Can you work these out from the drawing? Everything is in mm from the part's minimum corner. Round coordinates to 2 decimals unless told otherwise and drop trailing zeros. Loops run counter-clockwise (first coordinate to the right, second up) from the corner with the lowest first, then second, coordinate; pieces in that order, holes last. Notation, with made-up numbers: (27.5, 53) - (66.5, 53) arc R13 ccw to (66.5, 58) - close; hole circle Ø9 at (-38.75, -20). An arc over 180 degrees is marked (long way). Put each result on its own line as item: value. Start each with the question number.
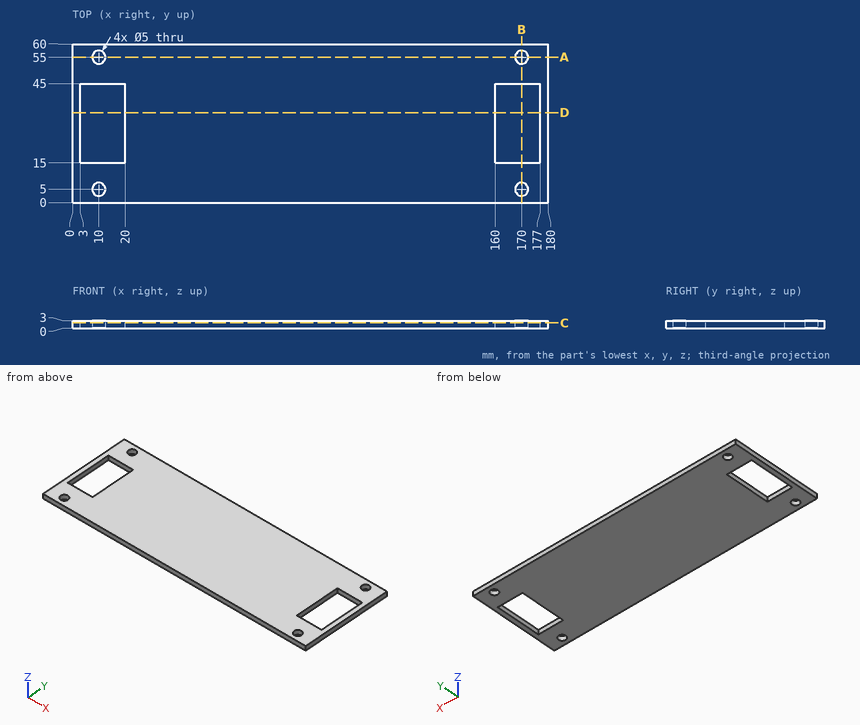
Item 1: Will this pin go through, and if not, where does the flat tip stop? P1, Ø4.5, axis at x = 170, y = 55, coming from the +Z side (3 decimals).
Item 2: I need wall thicknesses on line 1 (X direction, y = 19, z = 1.05); line 2 (Y direction, x = 170, z = 1.1); line 3 (X direction, y = 4, z = 0.85). Which ranges of each line are inside material? Lowest first, please. Write a range as from..to.
Item 3: Suppose I cut it at C-C, the plane z = 2.1. List the corners of the cut face in (x, y) for me, then the cut area to 3 significant figures.
Item 4: Suppose I cut it at D-D, the plane y = 34. List the corners of the cut face in (x, z) for me.
Item 5: Suppose I cut it at A-A, the plane y = 55. List the corners of the cut face in (x, z) for me.
Item 6: Suppose I cut it at B-B, the plane x = 170. List the corners of the cut face in (y, z) for me.
Numbers:
1. P1: through
2. line 1: 0..3, 20..160, 177..180
2. line 2: 0..2.5, 7.5..15, 45..52.5, 57.5..60
2. line 3: 0..7.71, 12.29..167.71, 172.29..180
3. outline: (0, 0) - (180, 0) - (180, 60) - (0, 60) - close; hole (3, 15) - (20, 15) - (20, 45) - (3, 45) - close; hole circle Ø5 at (10, 5); hole circle Ø5 at (10, 55); hole (160, 15) - (177, 15) - (177, 45) - (160, 45) - close; hole circle Ø5 at (170, 5); hole circle Ø5 at (170, 55)
3. area: 9,700 mm^2
4. outline: (0, 0) - (3, 0) - (3, 3) - (0, 3) - close; (20, 0) - (160, 0) - (160, 3) - (20, 3) - close; (177, 0) - (180, 0) - (180, 3) - (177, 3) - close
5. outline: (0, 0) - (7.5, 0) - (7.5, 3) - (0, 3) - close; (12.5, 0) - (167.5, 0) - (167.5, 3) - (12.5, 3) - close; (172.5, 0) - (180, 0) - (180, 3) - (172.5, 3) - close
6. outline: (0, 0) - (2.5, 0) - (2.5, 3) - (0, 3) - close; (7.5, 0) - (15, 0) - (15, 3) - (7.5, 3) - close; (45, 0) - (52.5, 0) - (52.5, 3) - (45, 3) - close; (57.5, 0) - (60, 0) - (60, 3) - (57.5, 3) - close
